Part model, mm, in its own coordinate system. A direction names the side the tool comes from. Coordinates: 2 decimals unless noted, no trailing zeros. Write each loop counter-clockwise with the first axis right and the second up, starting at its lowest first coordinate (ties: lowest second). Pieces come first, ordered by that corner, then holes. Notation, with made-up numbers: (57.25, -38) - (82.25, -38) arc R34 cw to (82.25, -8) - close; hole circle Ø11 at (71.25, 41). An arc over 180 degrees is marked (long way). Use a Markdown table: item, result.
```python
from build123d import *

# Parameters (mm, degrees)
SKETCH1_W           = 95
SKETCH1_H           = 95
SKETCH1_R           = 35.5
BOSS_EXTRUDE1_DEPTH = 2
SKETCH3_W           = 14
SKETCH3_H           = 4
SKETCH3_W_2         = 13
CUT_EXTRUDE5_DEPTH  = 68.294130502
SKETCH4_W           = 15
SKETCH4_H           = 4
BOSS_EXTRUDE2_DEPTH = 4
FILLET1_R           = 5


with BuildPart() as part:
    # Sketch1 → Boss-Extrude1 (new, symmetric)
    with BuildSketch(Plane(origin=(0, 0, 0), x_dir=(1, 0, 0), z_dir=(0, 1, 0))):
        Rectangle(SKETCH1_W, SKETCH1_H)
        with Locations(Location((0, 0, 0), (0, 0, 270))):
            Circle(SKETCH1_R, mode=Mode.SUBTRACT)
    extrude(amount=BOSS_EXTRUDE1_DEPTH, both=True)

    # Sketch3 → Cut-Extrude5 (cut, through all)
    with BuildSketch(Plane(origin=(0, 2, 0), x_dir=(1, 0, 0), z_dir=(0, 1, 0))):
        with Locations((-40.5, 37.5)):
            Rectangle(SKETCH3_W, SKETCH3_H)
        with Locations((-21, 37.5)):
            Rectangle(SKETCH3_W_2, SKETCH3_H)
        with Locations((21, 37.5)):
            Rectangle(SKETCH3_W_2, SKETCH3_H)
        with Locations((40.5, 37.5)):
            Rectangle(SKETCH3_W, SKETCH3_H)
        with Locations((40.5, -37.5)):
            Rectangle(SKETCH3_W, SKETCH3_H)
        with Locations((21, -37.5)):
            Rectangle(SKETCH3_W_2, SKETCH3_H)
        with Locations((-21, -37.5)):
            Rectangle(SKETCH3_W_2, SKETCH3_H)
        with Locations((-40.5, -37.5)):
            Rectangle(SKETCH3_W, SKETCH3_H)
    extrude(amount=-CUT_EXTRUDE5_DEPTH, mode=Mode.SUBTRACT)

    # Sketch4 → Boss-Extrude2 (add)
    with BuildSketch(Plane.ZY.offset(47.5)):
        with Locations((-18, 0)):
            Rectangle(SKETCH4_W, SKETCH4_H)
        with Locations((18, 0)):
            Rectangle(SKETCH4_W, SKETCH4_H)
    extrude(amount=BOSS_EXTRUDE2_DEPTH)

    # Fillet1
    fillet1_edges = [part.edges().sort_by_distance(p)[0] for p in [
        (47.5, 0, 47.5),
        (47.5, 0, -47.5),
    ]]
    fillet(fillet1_edges, radius=FILLET1_R)


solid = part.part
```
Item 1: Which spindle directions (+Z, -Z, +X, -X, +Y, -Y) get a long thin tool onto all of the face, cutting with end or side? Do faces 1 (the face through (-33.5, 0, 38)), 2 (the face through (-27.5, 0, -37)), 3 (the face through (-49, 0, -25.5)), 4 (the face through (40, 0, -39.5)). Say none if no direction does.
From the geometry:
| item | result |
|---|---|
| face 1 | -X, +Y, -Y |
| face 2 | +Y, -Y |
| face 3 | -Z, -X, +Y, -Y |
| face 4 | +X, +Y, -Y |
Item 2: Drill centre lines: probe 1 along Z at (x, y) = (-41, -0.05); probe 2 along X at (y, z) = (-1.3, 38); probe 3 along X at (y, z) = (-1.2, 0). Where is each one in solid material? Low to high.
From the geometry:
| item | result |
|---|---|
| probe 1 | -47.5 to -39.5, -35.5 to 35.5, 39.5 to 47.5 |
| probe 2 | -33.5 to -27.5, -14.5 to 14.5, 27.5 to 33.5 |
| probe 3 | -47.5 to -35.5, 35.5 to 47.5 |
Item 3: Band-saw the part on B-B, the plane z = 0. Give the cut face in (x, y), then the cut area to 3 significant figures.
From the geometry:
| item | result |
|---|---|
| outline | (-47.5, -2) - (-35.5, -2) - (-35.5, 2) - (-47.5, 2) - close; (35.5, -2) - (47.5, -2) - (47.5, 2) - (35.5, 2) - close |
| area | 96.0 mm^2 |
Item 4: Band-saw the part on C-C, the plane x = -37.5. Give the cut face in (y, z), then the cut area to 3 significant figures.
From the geometry:
| item | result |
|---|---|
| outline | (-2, -47.5) - (2, -47.5) - (2, -39.5) - (-2, -39.5) - close; (-2, -35.5) - (2, -35.5) - (2, 35.5) - (-2, 35.5) - close; (-2, 39.5) - (2, 39.5) - (2, 47.5) - (-2, 47.5) - close |
| area | 348 mm^2 |
Item 5: Band-saw the part on D-D, the plane y = -1.35. Count the separate pieces of the cut face and the enclosed holes in it, then the cut area to 3 significant figures.
From the geometry:
| item | result |
|---|---|
| separate pieces | 1 |
| enclosed holes | 5 |
| area | 4,740 mm^2 |
Item 6: Band-saw the part on A-A, the plane x = 0. Give the cut face in (y, z).
From the geometry:
| item | result |
|---|---|
| outline | (-2, -47.5) - (2, -47.5) - (2, -35.5) - (-2, -35.5) - close; (-2, 35.5) - (2, 35.5) - (2, 47.5) - (-2, 47.5) - close |
Item 7: Drop flat-ended pins along their axis: P1, Ø1.2, axis at y = 0, z = -37, coming from the -X side; P2, Ø2, axis at y = 1.5, z = 33, coming from the -X side. Give the stop position or say it passes through.
From the geometry:
| item | result |
|---|---|
| P1 | x = -33.5 |
| P2 | x = -47.5 |
Item 8: Two-plate mould, pull along X, no slides. Class faces 5 (the face through (-21, 0, -39.5)), 6 (the face through (-49, 0, 25.5)), 7 (the face through (33.5, 0, -37)): pulls with the +X half, pulls with the -X half, needs draft (parallel to the pull), parting line crosses it, or undercut.
From the geometry:
| item | result |
|---|---|
| face 5 | undercut |
| face 6 | needs draft |
| face 7 | pulls with the +X half |
